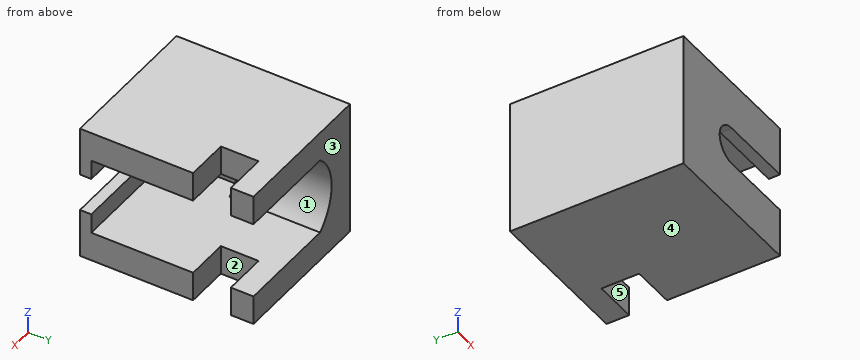
Autodesk Fusion 360 part; units mm, degrees
sketch "Sketch1" plane through (0, 0, 0) normal (0, 1, 0) x (1, 0, 0)
  line L0 (-10, -9) -> (10, -9)
  line L1 (10, -9) -> (10, 9)
  line L2 (10, 9) -> (-10, 9)
  line L3 (-10, 9) -> (-10, -9)
  line L4 (-10, 0) -> (10, 0) construction
  line L5 (0, 9) -> (0, -9) construction
  dimension "d1" = 18
  dimension "d2" = 20
extrude "Extrude1" add sketch "Sketch1" along normal blind 23
sketch "Sketch2" plane through (0, 0, 0) normal (0, -1, 0) x (1, 0, 0)
  line L0 (-10, 9) -> (-10, -9)
  line L1 (-10, -9) -> (10, -9)
  line L2 (10, -9) -> (10, 9)
  line L3 (10, 9) -> (-10, 9)
  line L4 (10, 2.5) -> (0, 2.5)
  line L5 (10, -2.5) -> (0, -2.5)
  arc A0 (0, 2.5) -> (0, -2.5) centre (0, 0) ccw
  line L6 (10, 2.5) -> (10, -2.5)
  dimension "d5" = 2.5
extrude "Extrude2" cut sketch "Sketch2" against normal blind 1.5 contours L2 L4 L5 A0 L6
sketch "Sketch3" plane through (0, 1.5, 0) normal (0, -1, 0) x (1, 0, 0)
  arc A0 (0, 2.5) -> (0, -2.5) centre (0, 0) ccw
  line L0 (0, -2.5) -> (10, -2.5)
  line L1 (10, -2.5) -> (10, 2.5)
  line L2 (10, 2.5) -> (0, 2.5)
  line L3 (10, 5.1) -> (-6.2, 5.1)
  line L4 (-6.2, 5.1) -> (-6.2, -5.1)
  line L5 (-6.2, -5.1) -> (10, -5.1)
  line L6 (10, -5.1) -> (10, 5.1)
  line L7 (-6.2, 0) -> (10, 0) construction
  dimension "d9" = 10.2
  dimension "d10" = 6.2
extrude "Extrude3" cut sketch "Sketch3" against normal blind 9.5
sketch "Sketch4" plane through (0, 11, 0) normal (0, -1, 0) x (1, 0, 0)
  line L0 (10, -5.1) -> (10, 5.1)
  line L1 (10, 5.1) -> (-6.2, 5.1)
  line L2 (-6.2, 5.1) -> (-6.2, -5.1)
  line L3 (-6.2, -5.1) -> (10, -5.1)
  arc A0 (-3.8, 5.1) -> (-3.8, -5.1) centre (0.4187, 0) ccw
  line L4 (-3.8, 5.1) -> (10, 5.1)
  line L5 (10, -5.1) -> (-3.8, -5.1)
  dimension "d13" = 2.4
extrude "Extrude4" cut sketch "Sketch4" against normal through all contours L0 L1 L3 A0 L4 L5
sketch "Sketch6" plane through (0, 23, 0) normal (0, 1, 0) x (-1, 0, 0)
  line L0 (3.8, -5.1) -> (-10, -5.1)
  line L1 (-10, -5.1) -> (-10, -9)
  line L2 (-10, -9) -> (10, -9)
  line L3 (10, -9) -> (10, 9)
  line L4 (10, 9) -> (-10, 9)
  line L5 (-10, 9) -> (-10, 5.1)
  line L6 (-10, 5.1) -> (3.8, 5.1)
  arc A0 (3.8, -5.1) -> (3.8, 5.1) centre (-0.4187, 0) ccw
  line L7 (-10, 9) -> (-4.25, 9)
  line L8 (-4.25, 9) -> (-4.25, 5.1)
  line L9 (-4.25, 5.1) -> (-10, 5.1)
  line L10 (-10, 5.1) -> (-10, 9)
  line L11 (-2.5, 0) -> (-20, 0)
  line L12 (-4.25, -9) -> (-4.25, -5.1)
  line L13 (-10, -9) -> (-4.25, -9)
  line L14 (-10, -5.1) -> (-10, -9)
  line L15 (-4.25, -5.1) -> (-10, -5.1)
  dimension "d17" = 5.75
extrude "Extrude5" cut sketch "Sketch6" against normal blind 5 from surface at -3 contours L0 L1 L2 L12 L13 L14 L15 | L4 L5 L6 L7 L8 L9 L10
Verification items for the finished model (mm, model axes). Face numbers are marked on the shaded views. A direction names the side the tool comes from. Round coordinates to 2 decimals unless told otherwise and drop trailing zeros. Write each loop counter-clockwise with the first axis right and the second up, starting at its lowest first coordinate (ties: lowest second). Pieces come first, ordered by that corner, then holes. Notation, with made-up numbers: (28.25, -8) - (56.25, -8) arc R19 cw to (56.25, 18) - close; hole circle Ø5 at (50, -37.75). An arc over 180 degrees is marked (long way). Answer as a JSON object with one key per item and string values. Group by question number.
Q1. Go/stop test with flat-tipped pins: pin 1 Ø4 at (x, z) = (2.5, -5) entering from -Y; pin 2 Ø5 at (y, z) = (5.5, 2.5) entering from +X; pin 3 Ø3 at (y, z) = (17.5, 8) entering from +X; pin 4 Ø2 at (x, z) = (7, -0.5) entering from -Y. Record where each tip stops, or that it passes through.
Q2. Mould release check, pull along Y, two halves, no side actions. Record for the marked faces 1, 2 and 3: released by +Y, released by -Y, zero draft, split by the parting line, or undercut.
Q3. Thickness scan on line 1 (Z direction, x = -1.25, y = 18.5); line 2 (Y direction, x = 5, z = -7.5); line 3 (Y direction, x = -5.75, z = 3.75). Record the ranges inside material, lowest first.
Q4. Section check A-A, the plane z = 7. Enter the section's corners in (x, y), plus the area to 3 significant figures.
Q5. Section check B-B, the plane y = 5. Enter the section's corners in (x, z).
Q6. Tool access check on the marked faces 4 and 5. Record the directions out of +Z, -Z, +X, -X, +Y, -Y that give a thin tool (end or side, any length) a straight path to the whole face; none if there is none.
Found:
{
 "1": {"pin 1": "stops at y = 0", "pin 2": "stops at x = -6.2", "pin 3": "stops at x = 4.25", "pin 4": "passes through"},
 "2": {"face 1": "zero draft", "face 2": "undercut", "face 3": "released by +Y"},
 "3": {"line 1": "z = -9 to -5.1, 5.1 to 9", "line 2": "y = 0 to 15, 20 to 23", "line 3": "y = 0 to 1.5, 11 to 23"},
 "4": {"outline": "(-10, 0) - (10, 0) - (10, 15) - (4.25, 15) - (4.25, 20) - (10, 20) - (10, 23) - (-10, 23) - close", "area": "431 mm^2"},
 "5": {"outline": "(-10, -9) - (10, -9) - (10, -5.1) - (-6.2, -5.1) - (-6.2, 5.1) - (10, 5.1) - (10, 9) - (-10, 9) - close"},
 "6": {"face 4": "-Z, +X, -X, +Y, -Y", "face 5": "+Z, -Z, +X"}
}
